Design review of the part built by this model. Coordinates are the model's own, in mm. Give positions to 0.01 mm unless a question says otherwise; leave off trailing zeros. Loops run counter-clockwise (first coordinate to the right, second up) from the corner with the lowest first, then second, coordinate; pieces in that order, holes last. Notation, with made-up numbers: (-6.5, 46.5) -> (27.5, 46.5) arc R8 ccw to (27.5, 58.5) -> close; hole circle Ø11 at (43, 33.5). An arc over 180 degrees is marked (long way). Use a Markdown table: item, result. Add a question column.
1. For pin 1 Ø6.5 at (x, y) = (-85, 35.21) entering from +Z; pin 2 Ø3.5 at (x, y) = (35.21, -85) entering from -Z; pin 3 Ø1 at (y, z) = (45, 2.5) entering from -X; pin 4 Ø1 at (y, z) = (77.5, 2) entering from -X, all flat-tipped, find the tip position at first contact; note any pin that passes through.
2. Add section A-A (y = 0). State the section outline as (x, z) points.
3. Add section B-B (z = 2.1). Count the separate pieces of the cut face and the enclosed holes in it, and give its area (3 significant figures).
4. Draft analysis for pull direction Y (two halves, no side actions). For faces 1 (the cylindrical face through (80, 0.6, 1.5)), 2 (the flat face through (-7, 1, 3)), 3 (the cylindrical face through (-99.932, 3.679, 1.479)), state which applies: pulls with the +Y half, pulls with the -Y half, needs draft (parallel to the pull), parting line crosses it, or undercut.
5. To check wall thickness, follow line 1 (X direction, y = -83.5, z = 1.4) (3 decimals); line 2 (X direction, y = 86.5, z = 0.75); line 3 (Y direction, x = 71, z = 2.9). State the ranges of each line that lie inside material, in increasing order.
6. Add section C-C (x = -57). State the section outline as (y, z) points.
```python
from build123d import *

# Parameters (mm, degrees)
CROQUIS1_R              = 100
SALIENTE_EXTRUIR1_DEPTH = 3
CROQUIS3_R              = 110
CORTAR_EXTRUIR1_DEPTH   = 3
REDONDEO1_R             = 10
CROQUIS4_R              = 2
CORTAR_EXTRUIR2_DEPTH   = 142.453172607


with BuildPart() as part:
    # Croquis1 → Saliente-Extruir1 (new body)
    with BuildSketch(Plane.XY):
        Circle(CROQUIS1_R)
    extrude(amount=SALIENTE_EXTRUIR1_DEPTH)

    # Croquis3 → Cortar-Extruir1 (cut)
    with BuildSketch(Plane.XY.offset(3)):
        with Locations((190, 0)):
            Circle(CROQUIS3_R)
    extrude(amount=-CORTAR_EXTRUIR1_DEPTH, mode=Mode.SUBTRACT)

    # Redondeo1
    redondeo1_edges = [part.edges().sort_by_distance(p)[0] for p in [
        (89.473684211, -44.659375654, 1.5),
        (89.473684211, 44.659375654, 1.5),
    ]]
    fillet(redondeo1_edges, radius=REDONDEO1_R)

    # Croquis4 → Cortar-Extruir2 (cut, through all)
    with BuildSketch(Plane(origin=(0, 0, 0), x_dir=(-1, 0, 0), z_dir=(0, 0, -1))):
        with Locations((-35.206875778, 84.996916991)):
            Circle(CROQUIS4_R)
        with Locations((35.206875778, 84.996916991)):
            Circle(CROQUIS4_R)
        with Locations((84.996916991, 35.206875778)):
            Circle(CROQUIS4_R)
        with Locations((84.996916991, -35.206875778)):
            Circle(CROQUIS4_R)
        with Locations((35.206875778, -84.996916991)):
            Circle(CROQUIS4_R)
        with Locations((-35.206875778, -84.996916991)):
            Circle(CROQUIS4_R)
    extrude(amount=-CORTAR_EXTRUIR2_DEPTH, mode=Mode.SUBTRACT)


solid = part.part
```
Taken from the geometry:
| question | item | result |
|---|---|---|
| 1 | pin 1 | stops at z = 3 |
| 1 | pin 2 | passes through |
| 1 | pin 3 | stops at x = -89.55 |
| 1 | pin 4 | stops at x = -63.8 |
| 2 | outline | (-100, 0) -> (80, 0) -> (80, 3) -> (-100, 3) -> close |
| 3 | separate pieces | 1 |
| 3 | enclosed holes | 6 |
| 3 | area | 30,100 mm^2 |
| 4 | face 1 | undercut |
| 4 | face 2 | needs draft |
| 4 | face 3 | parting line crosses it |
| 5 | line 1 | x = -55.025 to -36.533, -33.881 to 33.881, 36.533 to 55.025 |
| 5 | line 2 | x = -50.18 to -36.53, -33.89 to 33.89, 36.53 to 50.18 |
| 5 | line 3 | y = -70.42 to 70.42 |
| 6 | outline | (-82.16, 0) -> (82.16, 0) -> (82.16, 3) -> (-82.16, 3) -> close |
